from build123d import *

# Parameters (mm, degrees)
SKETCH2_W                = 25
SKETCH2_H                = 25
BOSS_EXTRUDE1_DEPTH      = 25
LPATTERN1_COUNT          = 2
LPATTERN1_PITCH          = 15
LPATTERN1_COUNT_DIR2     = 2
LPATTERN1_PITCH_DIR2     = 15
SKETCH6_R                = 4
BOSS_EXTRUDE3_DEPTH      = 5
BOSS_EXTRUDE3_DEPTH_BACK = 5
FILLET4_R                = 10


with BuildPart() as part:
    # Sketch2 → Boss-Extrude1 (new body)
    with BuildSketch(Plane(origin=(0, 0, 0), x_dir=(1, 0, 0), z_dir=(0, 1, 0))):
        Rectangle(SKETCH2_W, SKETCH2_H)
    extrude(amount=BOSS_EXTRUDE1_DEPTH)

    # Sketch4 → CSK for M3 Oval Head Machine Screw1 (revolve, cut)
    with BuildSketch(Plane(origin=(-12.5, 20, -7.5), x_dir=(0, 0, 1), z_dir=(0, 1, 0))):
        Polygon((0, 0), (0, 11.502151548), (2.5, 10), (2.5, 2.860133251), (2.7, 0), align=None)
    csk_for_m3_oval_head_machine_screw1 = revolve(axis=Axis((-18.85, 20, -7.5), (1, 0, 0)), mode=Mode.SUBTRACT)

    # LPattern1: CSK for M3 Oval Head Machine Screw1 2 × 2
    with Locations(*[(0, -i * LPATTERN1_PITCH, j * LPATTERN1_PITCH_DIR2) for i in range(LPATTERN1_COUNT) for j in range(LPATTERN1_COUNT_DIR2) if (i, j) != (0, 0)]):
        add(csk_for_m3_oval_head_machine_screw1, mode=Mode.SUBTRACT)

    # Mirror1: CSK for M3 Oval Head Machine Screw1 across plane
    add(csk_for_m3_oval_head_machine_screw1.mirror(Plane(origin=(0, 0, 0), x_dir=(0, 0, 1), z_dir=(1, 0, 0))), mode=Mode.SUBTRACT)

    # Mirror1 copy 1 sketch → Mirror1 copy 1 (revolve, cut)
    with BuildSketch(Plane(origin=(12.5, 20, 7.5), x_dir=(0, 0, 1), z_dir=(0, 1, 0))):
        Polygon((0, 0), (0, -11.502151548), (2.5, -10), (2.5, -2.860133251), (2.7, 0), align=None)
    revolve(axis=Axis((18.85, 20, 7.5), (1, 0, 0)), mode=Mode.SUBTRACT)

    # Mirror1 copy 2 sketch → Mirror1 copy 2 (revolve, cut)
    with BuildSketch(Plane(origin=(12.5, 5, -7.5), x_dir=(0, 0, 1), z_dir=(0, 1, 0))):
        Polygon((0, 0), (0, -11.502151548), (2.5, -10), (2.5, -2.860133251), (2.7, 0), align=None)
    revolve(axis=Axis((18.85, 5, -7.5), (1, 0, 0)), mode=Mode.SUBTRACT)

    # Mirror1 copy 3 sketch → Mirror1 copy 3 (revolve, cut)
    with BuildSketch(Plane(origin=(12.5, 5, 7.5), x_dir=(0, 0, 1), z_dir=(0, 1, 0))):
        Polygon((0, 0), (0, -11.502151548), (2.5, -10), (2.5, -2.860133251), (2.7, 0), align=None)
    revolve(axis=Axis((18.85, 5, 7.5), (1, 0, 0)), mode=Mode.SUBTRACT)

    # Sketch6 → Boss-Extrude3 (add, two sides)
    with BuildSketch(Plane.XY) as boss_extrude3_sk:
        with BuildLine():
            ThreePointArc((4.918032787, 34.098360656), (0, 40), (-4.918032787, 34.098360656))
            Line((-4.918032787, 34.098360656), (-12.5, 25))
            Line((-12.5, 25), (12.5, 25))
            Line((12.5, 25), (4.918032787, 34.098360656))
        make_face()
        with Locations((0, 35)):
            Circle(SKETCH6_R, mode=Mode.SUBTRACT)
    extrude(amount=BOSS_EXTRUDE3_DEPTH)
    extrude(boss_extrude3_sk.sketch, amount=-BOSS_EXTRUDE3_DEPTH_BACK)

    # Fillet4
    fillet4_edges = [part.edges().sort_by_distance(p)[0] for p in [
        (-4.918032787, 34.098360656, 0),
        (4.918032787, 34.098360656, 0),
    ]]
    fillet(fillet4_edges, radius=FILLET4_R)


solid = part.part
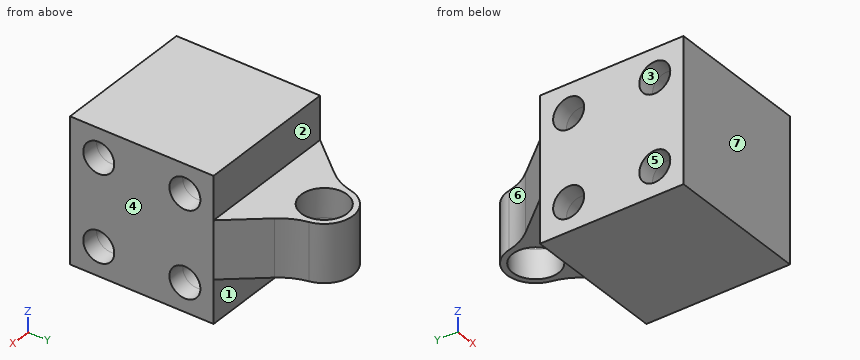
The model under review builds one solid part; all positions refer to its coordinate system, in mm. Face numbers are marked on the shaded views. A direction names the side the tool comes from. Coordinates: 2 decimals unless noted, no trailing zeros. Order: outer loops, then holes, each group sorted by start corner. A loop starts at its lowest first (then second) coordinate and runs counter-clockwise, first axis right, second up. Notation, with made-up numbers: (18, -39.5) -> (34, -39.5) arc R18 ccw to (34, -28.5) -> close; hole circle Ø5 at (-31, 1.25). An arc over 180 degrees is marked (long way). Answer in a Markdown table with one row per item.
(1) Insertion check: pin 1 (12 mm diameter, centred on x = 3, y = 36, fed in from -Z); pin 2 (9 mm diameter, centred on x = 0, y = 35, fed in from +Z); pin 3 (8 mm diameter, centred on x = 2.5, z = -10, fed in from +Y). Each pin has a flat end and moves straight along its axis. Give the tip position at first contact, or say it passes through.
Answers:
| item | result |
|---|---|
| pin 1 | z = -5 |
| pin 2 | z = 5 |
| pin 3 | y = 25 |
(2) Consider section B-B (z = -3.75). Write out the cut boundary in (x, y).
Answers:
| item | result |
|---|---|
| outline | (-12.5, 0) -> (12.5, 0) -> (12.5, 25) -> (7.02, 31.58) arc R10 cw to (4.9, 35.99) arc R5 ccw to (-4.9, 35.99) arc R10 cw to (-7.02, 31.58) -> (-12.5, 25) -> close; hole circle Ø8 at (0, 35) |
(3) Wall thickness on line 1 along Y through (x, z) = (4, -7.5); line 2 along Z through (x, y) = (5.25, 5); line 3 along Y through (x, z) = (3.5, -8.5): over which ranges is each line inside the solid? List them lowest first.
Answers:
| item | result |
|---|---|
| line 1 | 0 to 2.5, 7.5 to 17.5, 22.5 to 25 |
| line 2 | -12.5 to -10, -5 to 5, 10 to 12.5 |
| line 3 | 0 to 2.71, 7.29 to 17.71, 22.29 to 25 |
(4) The part is to be moulded in two halves that separate along Y. For the marked faces 4, 5, 6 and 7, say which applies: +Y half, -Y half, draft (parallel to the pull), parting line (faces both ways), or undercut.
Answers:
| item | result |
|---|---|
| face 4 | draft |
| face 5 | undercut |
| face 6 | +Y half |
| face 7 | -Y half |
(5) Machinability: for the marked faces 1, 2 and 3, which of the approach directions +Z, -Z, +X, -X, +Y, -Y give a long, thin tool a straight path to every point of the face, cutting with its end or side? Answer none if there is none.
Answers:
| item | result |
|---|---|
| face 1 | -Z, +X, -X, +Y |
| face 2 | +Z, +X, -X, +Y |
| face 3 | -X |
(6) Consider section C-C (y = 36.5). Write out the cut boundary in (x, z), plus the area to 3 significant figures.
Answers:
| item | result |
|---|---|
| outline | (-4.77, -5) -> (-3.71, -5) -> (-3.71, 5) -> (-4.77, 5) -> close; (3.71, -5) -> (4.77, -5) -> (4.77, 5) -> (3.71, 5) -> close |
| area | 21.2 mm² |
(7) Consider section D-D (x = 8.25). Write out the cut boundary in (y, z).
Answers:
| item | result |
|---|---|
| outline | (0, -12.5) -> (25, -12.5) -> (25, -5) -> (30.1, -5) -> (30.1, 5) -> (25, 5) -> (25, 12.5) -> (0, 12.5) -> close; hole circle Ø5 at (5, -7.5); hole circle Ø5 at (5, 7.5); hole circle Ø5 at (20, -7.5); hole circle Ø5 at (20, 7.5) |
(8) Consider section A-A (x = 0). Write out the cut boundary in (y, z).
Answers:
| item | result |
|---|---|
| outline | (0, -12.5) -> (25, -12.5) -> (25, -5) -> (31, -5) -> (31, 5) -> (25, 5) -> (25, 12.5) -> (0, 12.5) -> close; (39, -5) -> (40, -5) -> (40, 5) -> (39, 5) -> close |
